from build123d import *

# Parameters (mm, degrees)
F0_R     = 1.4
F1_DEPTH = 4.5
F2_R     = 3
F3_R     = 20


with BuildPart() as f1:
    # F0 (on Front) → F1 (new body)
    with BuildSketch(Plane.XZ):
        Polygon((-23.1, -38.3), (23.1, -38.3), (23.1, 38.3), (3.9, 38.3), (3.9, -21.7), (-3.9, -21.7), (-3.9, 38.3), (-23.1, 38.3), align=None)
        with Locations((-18.5, -16)):
            Circle(F0_R, mode=Mode.SUBTRACT)
        with Locations((18.5, -16)):
            Circle(F0_R, mode=Mode.SUBTRACT)
        with Locations((-18.5, 0)):
            Circle(F0_R, mode=Mode.SUBTRACT)
        with Locations((-18.5, 33.7)):
            Circle(F0_R, mode=Mode.SUBTRACT)
        with Locations((18.5, 0)):
            Circle(F0_R, mode=Mode.SUBTRACT)
        with Locations((18.5, 33.7)):
            Circle(F0_R, mode=Mode.SUBTRACT)
    extrude(amount=F1_DEPTH)

    # F2
    f2_edges = [f1.edges().sort_by_distance(p)[0] for p in [
        (-23.1, -2.25, 38.3),
        (23.1, -2.25, 38.3),
        (-3.9, -2.25, -21.7),
        (3.9, -2.25, -21.7),
        (-3.9, -2.25, 38.3),
        (3.9, -2.25, 38.3),
    ]]
    fillet(f2_edges, radius=F2_R)

    # F3
    f3_edges = [f1.edges().sort_by_distance(p)[0] for p in [
        (-23.1, -2.25, -38.3),
        (23.1, -2.25, -38.3),
    ]]
    fillet(f3_edges, radius=F3_R)


solid = f1.part
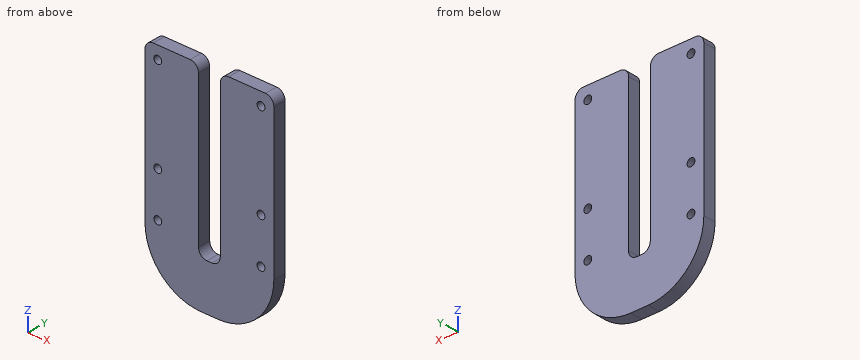
Geometry check sheet. Reference: the model listing, model coordinates, mm. Round coordinates to 2 decimals unless told otherwise and drop trailing zeros. Order: outer loops, then holes, each group sorted by start corner. A loop starts at its lowest first (then second) coordinate and runs counter-clockwise, first axis right, second up. Notation, with made-up numbers: (37, -37) - (61, -37) arc R21 cw to (61, -31) - close; hole circle Ø5 at (68.5, 37). An arc over 180 degrees is marked (long way). One line per question, with ' | ' between items. Start each with the question number.
(1) Sectioned sample at A-A on z = -12. Record the cut outline in (x, y), and give its area (3 significant figures).
(2) Sectioned sample at B-B on y = -3.4. Record the cut outline in (x, z).
(3) Thickness scan on L1, parallel to Z at x = -19, y = -3.6; L2, parallel to X at y = -2.2, z = -18; L3, parallel to Z at x = -18.5, y = -3.4. Record the ranges inside material, lowest first. Write a range as [from, to].
(4) Sectioned sample at D-D on x = 18.5. Record the cut outline in (y, z), and give its area (3 significant figures).
(5) Sectioned sample at C-C on z = 33.7. Record the cut outline in (x, y).
(6) Depth check by flat-ended pin: pin 1 Ø4.5 at (x, z) = (18.5, 33.7) entering from -Y; pin 2 Ø4 at (x, z) = (0, 28) entering from +Y (3 decimals); pin 3 Ø1 at (x, y) = (4.5, -2) entering from +Z; pin 4 Ø2 at (x, y) = (3.5, -3.5) entering from +Z. Enter the tip coordinate at first touch or a pass-through.
Conclusion:
1) outline: (-23.1, -4.5) - (-3.9, -4.5) - (-3.9, 0) - (-23.1, 0) - close; (3.9, -4.5) - (23.1, -4.5) - (23.1, 0) - (3.9, 0) - close | area: 173 mm2
2) outline: (-23.1, -18.3) arc R20 ccw to (-3.1, -38.3) - (3.1, -38.3) arc R20 ccw to (23.1, -18.3) - (23.1, 35.3) arc R3 ccw to (20.1, 38.3) - (6.9, 38.3) arc R3 ccw to (3.9, 35.3) - (3.9, -18.7) arc R3 cw to (0.9, -21.7) - (-0.9, -21.7) arc R3 cw to (-3.9, -18.7) - (-3.9, 35.3) arc R3 ccw to (-6.9, 38.3) - (-20.1, 38.3) arc R3 ccw to (-23.1, 35.3) - close; hole circle Ø2.8 at (-18.5, -16); hole circle Ø2.8 at (-18.5, 0); hole circle Ø2.8 at (-18.5, 33.7); hole circle Ø2.8 at (18.5, -16); hole circle Ø2.8 at (18.5, 0); hole circle Ø2.8 at (18.5, 33.7)
3) L1: z = [-30.43, -17.31], [-14.69, -1.31], [1.31, 32.39], [35.01, 38.3] | L2: x = [-23.1, -3.9], [3.9, 23.1] | L3: z = [-31.06, -17.4], [-14.6, -1.4], [1.4, 32.3], [35.1, 38.3]
4) outline: (-4.5, -31.06) - (0, -31.06) - (0, -17.4) - (-4.5, -17.4) - close; (-4.5, -14.6) - (0, -14.6) - (0, -1.4) - (-4.5, -1.4) - close; (-4.5, 1.4) - (0, 1.4) - (0, 32.3) - (-4.5, 32.3) - close; (-4.5, 35.1) - (0, 35.1) - (0, 38.3) - (-4.5, 38.3) - close | area: 274 mm2
5) outline: (-23.1, -4.5) - (-19.9, -4.5) - (-19.9, 0) - (-23.1, 0) - close; (-17.1, -4.5) - (-3.9, -4.5) - (-3.9, 0) - (-17.1, 0) - close; (3.9, -4.5) - (17.1, -4.5) - (17.1, 0) - (3.9, 0) - close; (19.9, -4.5) - (23.1, -4.5) - (23.1, 0) - (19.9, 0) - close
6) pin 1: stops at y = -4.5 | pin 2: passes through | pin 3: stops at z = 37.62 | pin 4: stops at z = 37.1
